from build123d import *

# Parameters (mm, degrees)
BOSS_EXTRUDE1_DEPTH    = 60
F_3DSKETCH1_R          = 1
CUT_EXTRUDE1_DEPTH     = 10
CUT_EXTRUDE3_OUTLINE_R = 12.5
CUT_EXTRUDE3_DEPTH     = 20
FILLET1_R              = 2
CUT_EXTRUDE4_DEPTH     = 60
FILLET2_R              = 2
CUT_EXTRUDE5_DEPTH     = 60
CUT_EXTRUDE8_START     = 16.42
CUT_EXTRUDE8_OUTLINE_R = 6.12
CUT_EXTRUDE8_DEPTH     = 3.58
CUT_EXTRUDE9_OUTLINE_R = 2.75
CUT_EXTRUDE9_DEPTH     = 16.42


# Read off the part's stored shape, not the designer's step: Cut-Extrude3, Cut-Extrude8, Cut-Extrude9
with BuildPart() as part:
    # Sketch1 → Boss-Extrude1 (new body)
    with BuildSketch(Plane.XY):
        Polygon((0, 0), (0, 80), (20, 80), (20, 20), (80, 20), (80, 0), align=None)
    extrude(amount=-BOSS_EXTRUDE1_DEPTH)

    # 3DSketch1 → Cut-Extrude1 (cut)
    with BuildSketch(Plane(origin=(20, 71.90061973, -50), x_dir=(0, -0.7071067811865477, 0.7071067811865475), z_dir=(-1, 0, 0))):
        with Locations(Location((0, 0, 0), (0, 0, 225))):
            Circle(F_3DSKETCH1_R)
        with Locations(Location((28.284271247, 28.284271247, 0), (0, 0, 225))):
            Circle(F_3DSKETCH1_R)
        with Locations(Location((27.881964101, -27.881964101, 0), (0, 0, 225))):
            Circle(F_3DSKETCH1_R)
        with Locations(Location((56.568542495, 0, 0), (0, 0, 225))):
            Circle(F_3DSKETCH1_R)
    extrude(amount=CUT_EXTRUDE1_DEPTH, mode=Mode.SUBTRACT)

    # Cut-Extrude3 outline → Cut-Extrude3 (cut)
    with BuildSketch(Plane.YZ):
        with Locations((50, -30)):
            Circle(CUT_EXTRUDE3_OUTLINE_R)
    extrude(amount=CUT_EXTRUDE3_DEPTH, mode=Mode.SUBTRACT)

    # Fillet1
    fillet1_edges = [part.edges().sort_by_distance(p)[0] for p in [
        (20, 37.5, -30),
        (0, 37.5, -30),
    ]]
    fillet(fillet1_edges, radius=FILLET1_R)

    # Sketch7 → Cut-Extrude4 (cut)
    with BuildSketch(Plane(origin=(80, 0, 0), x_dir=(0, 0, -1), z_dir=(1, 0, 0))):
        Polygon((0, 20), (2, 20), (0, 18), align=None)
        Polygon((60, 20), (58, 20), (60, 18), align=None)
    extrude(amount=-CUT_EXTRUDE4_DEPTH, mode=Mode.SUBTRACT)

    # Fillet2
    fillet2_edges = [part.edges().sort_by_distance(p)[0] for p in [
        (20, 20, -30),
    ]]
    fillet(fillet2_edges, radius=FILLET2_R)

    # Sketch8 → Cut-Extrude5 (cut)
    with BuildSketch(Plane.XY):
        Polygon((78, 20), (80, 20), (80, 18), align=None)
    extrude(amount=-CUT_EXTRUDE5_DEPTH, mode=Mode.SUBTRACT)

    # Cut-Extrude8 outline → Cut-Extrude8 (cut)
    with BuildSketch(Plane(origin=(0, 0, 0), x_dir=(1, 0, 0), z_dir=(0, 1, 0)).offset(CUT_EXTRUDE8_START)):
        with Locations((58, 48)):
            Circle(CUT_EXTRUDE8_OUTLINE_R)
    extrude(amount=CUT_EXTRUDE8_DEPTH, mode=Mode.SUBTRACT)

    # Cut-Extrude9 outline → Cut-Extrude9 (cut)
    with BuildSketch(Plane(origin=(0, 0, 0), x_dir=(1, 0, 0), z_dir=(0, 1, 0))):
        with Locations((58, 48)):
            Circle(CUT_EXTRUDE9_OUTLINE_R)
    extrude(amount=CUT_EXTRUDE9_DEPTH, mode=Mode.SUBTRACT)


solid = part.part
Work out the finished part from the listing and answer in its coordinate system (mm). A direction names the side the tool comes from. Round coordinates to 2 decimals unless told otherwise and drop trailing zeros. Loops run counter-clockwise (first coordinate to the right, second up) from the corner with the lowest first, then second, coordinate; pieces in that order, holes last. Notation, with made-up numbers: (-24.5, 39) - (30.5, 39) arc R32 cw to (30.5, 78) - close; hole circle Ø4 at (-14, 77). An arc over 180 degrees is marked (long way). One line per item, written item: value.
Q1. Find section A-A on z = -30. Give the vertices of the cut face in (x, y), and give its area (3 significant figures).
Check values:
outline: (0, 0) - (80, 0) - (80, 18) - (78, 20) - (22, 20) arc R2 cw to (20, 22) - (20, 35.5) arc R2 ccw to (18, 37.5) - (2, 37.5) arc R2 ccw to (0, 35.5) - close; (0, 64.5) arc R2 ccw to (2, 62.5) - (18, 62.5) arc R2 ccw to (20, 64.5) - (20, 80) - (0, 80) - close
area: 2,300 mm2
Q2. Straight lines are drawn through the part: probe 1 along Y at (x, z) = (16.25, -50); probe 2 along Y at (x, z) = (15, -10); probe 3 along X at (y, z) = (12.25, -48). For each, find the intervals that lie inside material, in ascending order.
Check values:
probe 1: 0 to 31.47, 33.47 to 70.9, 72.9 to 80
probe 2: 0 to 30.9, 32.9 to 70.9, 72.9 to 80
probe 3: 0 to 55.25, 60.75 to 80
Q3. Find section B-B on x = 58. Give the vertices of the cut face in (y, z), and give its area (3 significant figures).
Check values:
outline: (0, -60) - (18, -60) - (20, -58) - (20, -54.12) - (16.42, -54.12) - (16.42, -50.75) - (0, -50.75) - close; (0, -45.25) - (16.42, -45.25) - (16.42, -41.88) - (20, -41.88) - (20, -2) - (18, 0) - (0, 0) - close
area: 1,060 mm2
Q4. The mould has two halves that part along Z. Classify faces 1 (the flat face through (10, 72, -10)), 2 (the flat face through (50, 20, -30)), 3 (the flat face through (14, 23, 0)): +Z half, -Z half, draft (parallel to the pull), parting line (faces both ways), or undercut.
Check values:
face 1: undercut
face 2: draft
face 3: +Z half
Q5. Find section C-C on x = 70. Give the vertices of the cut face in (y, z), and give its area (3 significant figures).
Check values:
outline: (0, -60) - (18, -60) - (20, -58) - (20, -2) - (18, 0) - (0, 0) - close
area: 1,200 mm2
Q6. For faces 4 (the flat face through (59, 16.42, -45)), 5 (the cylindrical face through (15.07, 33.357, -50.461)), 6 (the flat face through (50, 19, -1)), 7 (the flat face through (50, 19, -59)), 8 (the cylindrical face through (20.57, 20.6, -30.39)), determine the directions among +Z, -Z, +X, -X, +Y, -Y from which every point of the face is accessible in a straight line to the end or side of a thin tool.
Check values:
face 4: +Y
face 5: +X
face 6: +Z, +X, +Y
face 7: -Z, +X, +Y
face 8: +Z, -Z, +X, +Y
Q7. Each of these flat-tipped pins is pushed along its axis until it touches: pin 1 Ø6 at (x, z) = (57, -51) entering from +Y; pin 2 Ø0.6 at (y, z) = (72, -10.5) entering from +X; pin 3 Ø1 at (y, z) = (59, -21) entering from +X; pin 4 Ø4.5 at (x, z) = (58, -48) entering from +Y. Where does it stop, or does it pass through?
Check values:
pin 1: y = 20
pin 2: x = 10
pin 3: x = 19.54
pin 4: through
